Can you work these out from the model? Positions are in its coordinate system, mm. Face numbers are marked on the shaded views. A direction names the side the tool comes from. Round coordinates to 2 decimals unless told otherwise and drop trailing zeros. Loops run counter-clockwise (first coordinate to the right, second up) from the corner with the lowest first, then second, coordinate; pieces in that order, holes last. Notation, with made-up numbers: M 31.25,22 L 43.25,22 A15 ccw 43.25,44 Z; hole C -13,-1 d3. An arc over 180 degrees is marked long. Use a Markdown table: item, result. Add a question column.
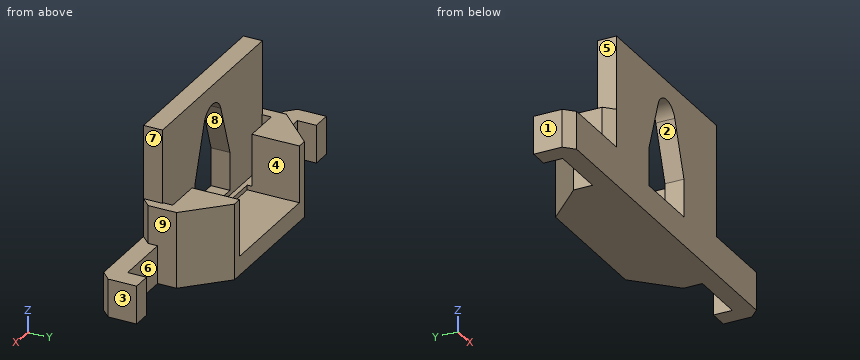
```python
from build123d import *

# Parameters (mm, degrees)
PAD012_DEPTH        = 10
SKETCH042_W         = 8
SKETCH042_H         = 1.125
PAD013_DEPTH        = 8
SKETCH043_W         = 6
SKETCH043_H         = 12
POCKET028_DEPTH     = 6
POCKET029_DEPTH     = 5
CHAMFER027_SIZE     = 1
CHAMFER028_SIZE     = 4
PAD014_DEPTH        = 4
CHAMFER029_SIZE     = 1
CLONE009_ROLL_ANGLE = -90


with BuildPart() as part:
    # Sketch041 → Pad012 (new body, symmetric)
    with BuildSketch(Plane.YZ):
        Polygon((-3.25, -21), (-3.25, -23), (12.5, -23), (12.5, -15), (4.5, -15), (4.5, -20), (10, -20), (10, -21), align=None)
    extrude(amount=PAD012_DEPTH, both=True)

    # Sketch042 → Pad013 (new body)
    with BuildSketch(Plane.YX.offset(23)):
        with Locations((8.5, 10.4375)):
            Rectangle(SKETCH042_W, SKETCH042_H)
    pad013 = extrude(amount=-PAD013_DEPTH)

    # Mirrored003: Pad013 across Sketch042 H_Axis
    add(pad013.mirror(Plane(origin=(0, 0, -23), x_dir=(0, 0, -1), z_dir=(1, 0, 0))))

    # Sketch043 → Pocket028 (cut)
    with BuildSketch(Plane(origin=(0, 4.5, 0), x_dir=(0, 0, -1), z_dir=(0, -1, 0))):
        with Locations((17.5, 0)):
            Rectangle(SKETCH043_W, SKETCH043_H)
    extrude(amount=-POCKET028_DEPTH, mode=Mode.SUBTRACT)

    # Sketch044 → Pocket029 (cut)
    with BuildSketch(Plane.YX.offset(23)):
        with BuildLine():
            Line((5.5, 3.5), (9.5, 3.5))
            Line((9.5, 3.5), (9.5, -3.5))
            Line((9.5, -3.5), (5.5, -3.5))
            Line((5.5, -3.5), (-0.050331, -1.661215))
            ThreePointArc((-0.050345, 1.661211), (-1.25, -7e-06), (-0.050331, -1.661215))
            Line((5.5, 3.5), (-0.050345, 1.661211))
        make_face()
    extrude(amount=-POCKET029_DEPTH, mode=Mode.SUBTRACT)

    # Chamfer027
    chamfer027_edges = [part.edges().sort_by_distance(p)[0] for p in [
        (11, 8.5, -23),
        (-11, 8.5, -23),
    ]]
    chamfer(chamfer027_edges, length=CHAMFER027_SIZE)

    # Chamfer028
    chamfer028_edges = [part.edges().sort_by_distance(p)[0] for p in [
        (-11, 8.5, -15),
        (11, 8.5, -15),
    ]]
    chamfer(chamfer028_edges, length=CHAMFER028_SIZE)

    # Sketch045 → Pad014 (new body)
    with BuildSketch(Plane.ZX.offset(12.5)):
        Polygon((-23, 9), (-21, 9), (-21, 17), (-19, 17), (-19, 19), (-23, 19), align=None)
    pad014 = extrude(amount=-PAD014_DEPTH)

    # Mirrored004: Pad014 across Sketch045 H_Axis
    add(pad014.mirror(Plane(origin=(0, 12.5, 0), x_dir=(0, 1, 0), z_dir=(1, 0, 0))))

    # Chamfer029
    chamfer029_edges = [part.edges().sort_by_distance(p)[0] for p in [
        (-19, 10.5, -23),
        (19, 10.5, -23),
    ]]
    chamfer(chamfer029_edges, length=CHAMFER029_SIZE)


with BuildPart() as part_1:
    # Clone009 roll: moved
    add(part.part.rotate(Axis((0, 0, 0), (1, 0, 0)), CLONE009_ROLL_ANGLE))


with BuildPart() as part_2:
    # Clone009 placement: moved
    add(part_1.part.moved(Location((-112, -13, -25.5))))


solid = part_2.part
```
(1) Suppose I cut it at C-C on x = -105.5. List the corners of the cut face in (y, z) for me, and give its area (3 significant figures).
(2) If I drill on probe 1 along Z at (x, y) = (-116.5, -31.75); probe 2 along Y at (x, z) = (-108.5, -24.75); probe 3 along X at (y, z) = (-32.75, -30.75), over which ranges is the centre line in solid material (lowest first)? Write a range as [from, to].
(3) On a 3-axis mill with a long thin cutter (end or side, diameter ignored), from which of +Z, -Z, +X, -X, +Y, -Y can I reach the whole of each face in a straight line? I mean the marked faces 5, 6, 7, 8 and 9. Say none if no direction works.
(4) Suppose I cut it at B-B on y = -28.5. List the corners of the cut face in (x, z) for me, and give its area (3 significant figures).
(5) Suppose I cut it at A-A on z = -33.25. List the corners of the cut face in (x, y) for me (3 decimals).
(6) I'm going to push flat-ended pins straight in: pin 1 (1.5 mm diameter, centred on x = -120, y = -30.5, fed in from +Z); pin 2 (1.6 mm diameter, centred on x = -109.5, y = -32, fed in from +Z); pin 3 (1.2 mm diameter, centred on x = -125, z = -36, fed in from +Y). Where does each tip first touch, or does it pass through?
(7) Suppose I cut it at D-D on x = -111. List the corners of the cut face in (y, z) for me.
(8) Thinking about a two-plate mould opening in X: for the marked faces 1, 2, 3 and 4, which applies, released by +X, released by -X, zero draft, split by the parting line, or undercut?
Results below:
| question | item | result |
|---|---|---|
| 1 | outline | M -36,-38 L -28,-38 L -28,-30 L -33,-30 L -33,-35.5 L -34,-35.5 L -34,-22.25 L -36,-22.25 Z |
| 1 | area | 74.0 mm² |
| 2 | probe 1 | z = [-38, -36] |
| 2 | probe 2 | y = [-36, -34] |
| 2 | probe 3 | x = [-123, -118], [-106, -101] |
| 3 | face 5 | +Z, -X, +Y, -Y |
| 3 | face 6 | +Z, -Z, +Y |
| 3 | face 7 | +Z, +X, +Y, -Y |
| 3 | face 8 | +Y, -Y |
| 3 | face 9 | +Z, +Y |
| 4 | outline | M -119.5,-38 L -104.5,-38 L -104.5,-30 L -106,-30 L -106,-36 L -118,-36 L -118,-30 L -119.5,-30 Z |
| 4 | area | 48.0 mm² |
| 5 | outline | M -123,-35 L -122,-36 L -115.5,-36 L -115.5,-34 L -121.875,-34 L -121.875,-33 L -118,-33 L -118,-28 L -119,-28 L -123,-32 Z; M -108.5,-36 L -102,-36 L -101,-35 L -101,-32 L -105,-28 L -106,-28 L -106,-33 L -102.125,-33 L -102.125,-34 L -108.5,-34 Z |
| 6 | pin 1 | stops at z = -30 |
| 6 | pin 2 | stops at z = -36 |
| 6 | pin 3 | stops at y = -34 |
| 7 | outline | M -36,-38 L -28,-38 L -28,-36 L -33.5,-36 L -33.5,-35.5 L -34,-35.5 L -34,-35 L -36,-35 Z; M -36,-24.56 L -34,-24.56 L -34,-22.25 L -36,-22.25 Z |
| 8 | face 1 | released by -X |
| 8 | face 2 | undercut |
| 8 | face 3 | released by +X |
| 8 | face 4 | undercut |
